Here's the drawing with two shaded views (mm, measured from the low corner). I have some questions. Round coordinates to 2 decimals unless told otherwise and drop trailing zeros. Loops run counter-clockwise (first coordinate to the right, second up) from the corner with the lowest first, then second, coordinate; pieces in that order, holes last.
(1) Will this pin go through, and if not, where does the flat tip stop? pin 1 Ø1 at (x, y) = (9, 7) entering from -Z.
(2) Thinking about a two-plate mould opening in X: for the marked faces 1, 2 and 3, which applies, released by +X, released by -X, zero draft, split by the parting line, or undercut?
(3) I want a section at A-A on y = 6. Write out the boundary of the cut face in (x, z).
(4) If I drill on line 1 along Y through (x, z) = (6, 2.7); line 2 along Y through (x, z) = (4.5, 2.7); line 3 along X through (y, z) = (9, 2.4), over which ranges is the centre line in solid material (lowest first)?
(5) I want a section at C-C on z = 0.4. Write out the boundary of the cut face in (x, y).
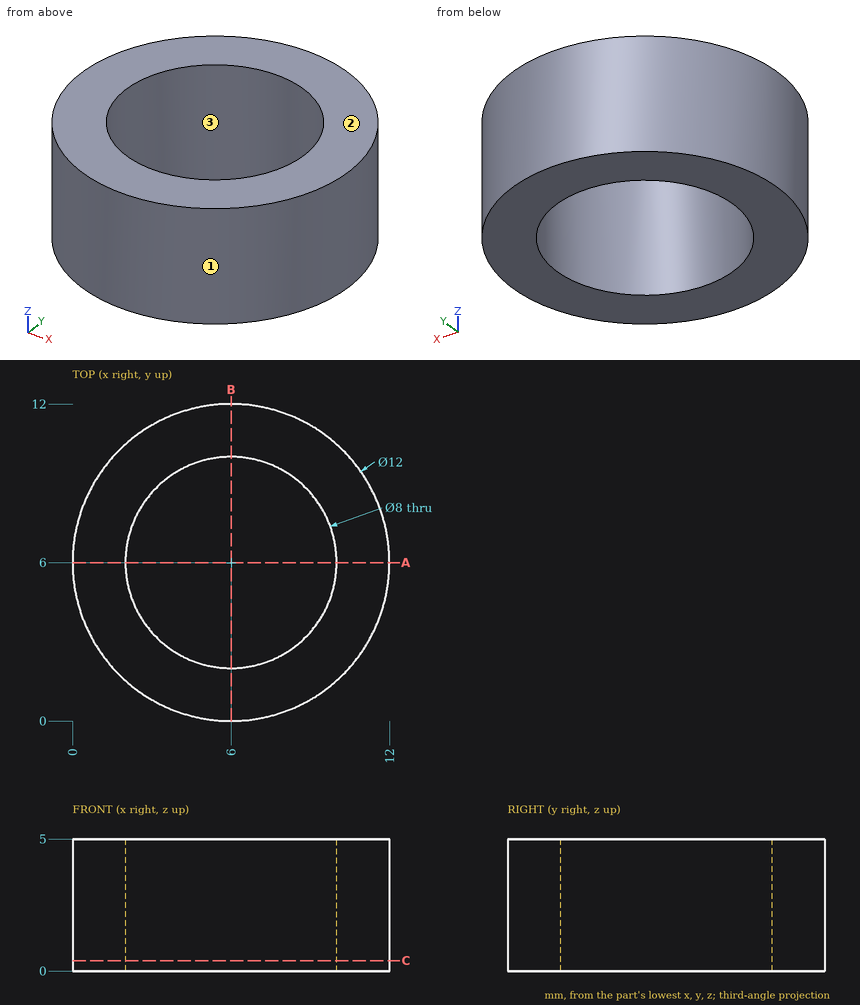
Filled sheet:
1. pin 1: passes through
2. face 1: split by the parting line
2. face 2: zero draft
2. face 3: undercut
3. outline: (0, 0) - (2, 0) - (2, 5) - (0, 5) - close; (10, 0) - (12, 0) - (12, 5) - (10, 5) - close
4. line 1: y = 0 to 2, 10 to 12
4. line 2: y = 0.19 to 2.29, 9.71 to 11.81
4. line 3: x = 0.8 to 3.35, 8.65 to 11.2
5. outline: circle Ø12 at (6, 6); hole circle Ø8 at (6, 6)
